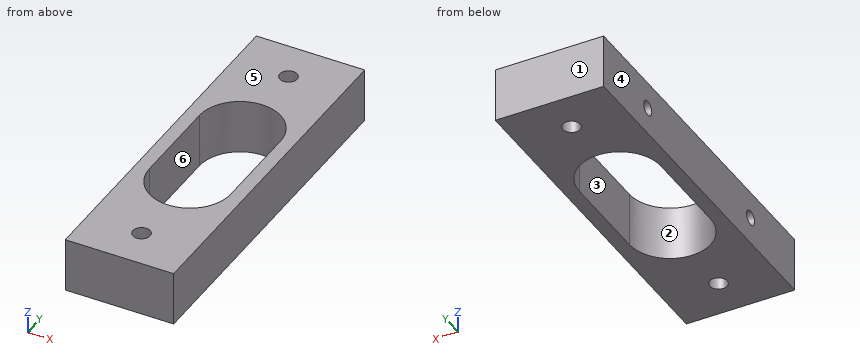
from build123d import *

# Parameters (mm, degrees)
SKETCH1_W                           = 25.4
SKETCH1_H                           = 12.7
BOSS_EXTRUDE1_DEPTH                 = 82.55
F_10_32_TAPPED_HOLE_TOP_HOLD_D      = 4.0386
F_8_32_TAPPED_HOLE_SIDE_PLATE_D     = 3.4544
F_8_32_TAPPED_HOLE_SIDE_PLATE_DEPTH = 12.2936
F_8_32_TAPPED_HOLE_SIDE_PLATE_TIP   = 1.037806461
CUT_EXTRUDE1_DEPTH                  = 88.298066989


with BuildPart() as part:
    # Sketch1 → Boss-Extrude1 (new body)
    with BuildSketch(Plane(origin=(0, 0, 0), x_dir=(1, 0, 0), z_dir=(0, 1, 0))):
        with Locations((12.7, 6.35)):
            Rectangle(SKETCH1_W, SKETCH1_H)
    extrude(amount=BOSS_EXTRUDE1_DEPTH)

    # #10-32 Tapped Hole - Top Hold (through all)
    with Locations(Plane(origin=(0, 0, -12.7), x_dir=(-1, 0, 0), z_dir=(0, 0, -1))):
        with Locations((-12.7, 9.525), (-12.7, 73.025)):
            Hole(F_10_32_TAPPED_HOLE_TOP_HOLD_D / 2)

    # #8-32 Tapped Hole - Side Plate
    with Locations(Plane.ZY):
        with Locations((-6.35, 19.05), (-6.35, 63.5)):
            Hole(F_8_32_TAPPED_HOLE_SIDE_PLATE_D / 2, depth=F_8_32_TAPPED_HOLE_SIDE_PLATE_DEPTH)
            with Locations((0, 0, -(F_8_32_TAPPED_HOLE_SIDE_PLATE_DEPTH + F_8_32_TAPPED_HOLE_SIDE_PLATE_TIP / 2))):  # 118° drill point
                Cone(0, F_8_32_TAPPED_HOLE_SIDE_PLATE_D / 2, F_8_32_TAPPED_HOLE_SIDE_PLATE_TIP, mode=Mode.SUBTRACT)

    # Sketch8 → Cut-Extrude1 (cut, through all)
    with BuildSketch(Plane(origin=(0, 0, -12.7), x_dir=(-1, 0, 0), z_dir=(0, 0, -1))):
        with BuildLine():
            Line((-22.225, 30.48), (-22.225, 52.07))
            ThreePointArc((-22.225, 52.07), (-12.7, 61.595), (-3.175, 52.07))
            Line((-3.175, 52.07), (-3.175, 30.48))
            ThreePointArc((-3.175, 30.48), (-12.7, 20.955), (-22.225, 30.48))
        make_face()
    extrude(amount=-CUT_EXTRUDE1_DEPTH, mode=Mode.SUBTRACT)


solid = part.part
CAD build for the part. Positions are in the model's coordinates, mm. Face numbers are marked on the shaded views. A direction names the side the tool comes from. Coordinates: 2 decimals unless noted, no trailing zeros. Order: outer loops, then holes, each group sorted by start corner. A loop starts at its lowest first (then second) coordinate and runs counter-clockwise, first axis right, second up. Notation, with made-up numbers: (42, 58) -> (59, 58) arc R22 ccw to (59, 64) -> close; hole circle Ø8 at (64, 47). An arc over 180 degrees is marked (long way). Answer in a Markdown table with one row per item.
1) Band-saw the part on C-C (x = 19). List the corners of the cut face in (y, z), and give its area (3 significant figures).
Check values:
| item | result |
|---|---|
| outline | (0, -12.7) -> (23.34, -12.7) -> (23.34, 0) -> (0, 0) -> close; (59.21, -12.7) -> (82.55, -12.7) -> (82.55, 0) -> (59.21, 0) -> close |
| area | 593 mm2 |
2) Which spindle directions (+Z, -Z, +X, -X, +Y, -Y) get a long thin tool onto all of the face, cutting with end or side? Do the marked faces 1 and 2. Say none if no direction does.
Check values:
| item | result |
|---|---|
| face 1 | +Z, -Z, +X, -X, +Y |
| face 2 | +Z, -Z |
3) Band-saw the part on A-A (y = 39). List the corners of the cut face in (x, z) (3 decimals).
Check values:
| item | result |
|---|---|
| outline | (0, -12.7) -> (3.175, -12.7) -> (3.175, 0) -> (0, 0) -> close; (22.225, -12.7) -> (25.4, -12.7) -> (25.4, 0) -> (22.225, 0) -> close |
4) Drill centre lines: line 1 (Y direction, x = 2.75, z = -6.35); line 2 (X direction, y = 52, z = -7.5) (3 decimals); line 3 (Y direction, x = 12.7, z = -6.25) (3 decimals). Where is each one in solid material? Low to high.
Check values:
| item | result |
|---|---|
| line 1 | 0 to 17.32, 20.78 to 61.77, 65.23 to 82.55 |
| line 2 | 0 to 3.175, 22.225 to 25.4 |
| line 3 | 0 to 7.506, 11.544 to 18.004, 20.096 to 20.955, 61.595 to 62.454, 64.546 to 71.006, 75.044 to 82.55 |
5) Flat gauge pin, fed straight in: P1, Ø3, axis at y = 19.05, z = -6.35, coming from the -X side. Where does the tip first touch, or does it go through?
Check values:
| item | result |
|---|---|
| P1 | x = 12.43 |
6) Mould opens along X. For the marked faces 3, 4, 5 and 6 say: pulls with the +X half, pulls with the -X half, needs draft (parallel to the pull), parting line crosses it, or undercut.
Check values:
| item | result |
|---|---|
| face 3 | undercut |
| face 4 | pulls with the -X half |
| face 5 | needs draft |
| face 6 | undercut |
7) Band-saw the part on B-B (x = 6). List the corners of the cut face in (y, z), and give its area (3 significant figures).
Check values:
| item | result |
|---|---|
| outline | (0, -12.7) -> (23.71, -12.7) -> (23.71, 0) -> (0, 0) -> close; (58.84, -12.7) -> (82.55, -12.7) -> (82.55, 0) -> (58.84, 0) -> close; hole circle Ø3.45 at (19.05, -6.35); hole circle Ø3.45 at (63.5, -6.35) |
| area | 583 mm2 |
8) Band-saw the part on D-D (z = -9.75). List the corners of the cut face in (x, y) (3 decimals), and give its area (3 significant figures).
Check values:
| item | result |
|---|---|
| outline | (0, 0) -> (25.4, 0) -> (25.4, 82.55) -> (0, 82.55) -> close; hole (3.175, 30.48) arc R9.525 ccw to (22.225, 30.48) -> (22.225, 52.07) arc R9.525 ccw to (3.175, 52.07) -> close; hole circle Ø4.039 at (12.7, 9.525); hole circle Ø4.039 at (12.7, 73.025) |
| area | 1,370 mm2 |
